from build123d import *

# Parameters (mm, degrees)
SM_BASE_FLANGE_1_DEPTH = 307.5
SKETCH_6_R             = 5.25
SKETCH_6_R_2           = 2.5
CUT_EXTRUDE_1_DEPTH    = 10
CUT_EXTRUDE_2_DEPTH    = 10
SKETCH_9_R             = 5.5
CUT_EXTRUDE_4_DEPTH    = 334.850640257
CHAMFER_1_SIZE         = 5


# Sheet-metal steps are written as plain solids
with BuildPart() as part:
    # Sketch 1 → Базовая кромка1 (new, symmetric)
    with BuildSketch(Plane.XY):
        with BuildLine():
            Line((-78, 64), (-78, 42))
            ThreePointArc((-78, 42), (-76.828427125, 39.171572875), (-74, 38))
            Line((-74, 38), (-2, 38))
            ThreePointArc((-2, 38), (-0.585786438, 37.414213562), (0, 36))
            Line((0, 36), (0, -36))
            ThreePointArc((0, -36), (-0.585786438, -37.414213562), (-2, -38))
            Line((-2, -38), (-74, -38))
            ThreePointArc((-74, -38), (-76.828427125, -39.171572875), (-78, -42))
            Line((-78, -42), (-78, -64))
            Line((-78, -64), (-76, -64))
            Line((-76, -64), (-76, -42))
            ThreePointArc((-76, -42), (-75.414213562, -40.585786438), (-74, -40))
            Line((-74, -40), (-2, -40))
            ThreePointArc((-2, -40), (0.828427125, -38.828427125), (2, -36))
            Line((2, -36), (2, 36))
            ThreePointArc((2, 36), (0.828427125, 38.828427125), (-2, 40))
            Line((-2, 40), (-74, 40))
            ThreePointArc((-74, 40), (-75.414213562, 40.585786438), (-76, 42))
            Line((-76, 42), (-76, 64))
            Line((-76, 64), (-78, 64))
        make_face()
    extrude(amount=SM_BASE_FLANGE_1_DEPTH, both=True)

    # Эскиз6 → Вырез-Вытянуть1 (cut)
    with BuildSketch(Plane(origin=(-76, 0, 0), x_dir=(0, 0, -1), z_dir=(1, 0, 0))):
        with Locations(Location((280, 55, 0), (0, 0, 90))):
            Circle(SKETCH_6_R)
        with Locations(Location((255, 55, 0), (0, 0, 90))):
            Circle(SKETCH_6_R)
        with Locations(Location((180, 57.5, 0), (0, 0, 90))):
            Circle(SKETCH_6_R_2)
        with Locations(Location((90, 57.5, 0), (0, 0, 90))):
            Circle(SKETCH_6_R_2)
        with Locations(Location((0, 57.5, 0), (0, 0, 90))):
            Circle(SKETCH_6_R_2)
        with Locations(Location((-90, 57.5, 0), (0, 0, 270))):
            Circle(SKETCH_6_R_2)
        with Locations(Location((-180, 57.5, 0), (0, 0, 270))):
            Circle(SKETCH_6_R_2)
        with Locations(Location((-255, 55, 0), (0, 0, 270))):
            Circle(SKETCH_6_R)
        with Locations(Location((-280, 55, 0), (0, 0, 270))):
            Circle(SKETCH_6_R)
    cut_extrude_1 = extrude(amount=-CUT_EXTRUDE_1_DEPTH, mode=Mode.SUBTRACT)

    # Зеркальное отражение1: Вырез-Вытянуть1 across plane
    add(cut_extrude_1.mirror(Plane.ZX), mode=Mode.SUBTRACT)

    # Эскиз7 → Вырез-Вытянуть2 (cut)
    with BuildSketch(Plane(origin=(2, 0, 0), x_dir=(0, 0, -1), z_dir=(1, 0, 0))):
        with BuildLine():
            Line((-288.5, 6.5), (-261.5, 6.5))
            ThreePointArc((-261.5, 6.5), (-255, 0), (-261.5, -6.5))
            Line((-261.5, -6.5), (-288.5, -6.5))
            ThreePointArc((-288.5, -6.5), (-295, 0), (-288.5, 6.5))
        make_face()
        with BuildLine():
            Line((-233.5, 6.5), (-206.5, 6.5))
            ThreePointArc((-206.5, 6.5), (-200, 0), (-206.5, -6.5))
            Line((-206.5, -6.5), (-233.5, -6.5))
            ThreePointArc((-233.5, -6.5), (-240, 0), (-233.5, 6.5))
        make_face()
        with BuildLine():
            Line((288.5, 6.5), (261.5, 6.5))
            ThreePointArc((261.5, 6.5), (255, 0), (261.5, -6.5))
            Line((261.5, -6.5), (288.5, -6.5))
            ThreePointArc((288.5, -6.5), (295, 0), (288.5, 6.5))
        make_face()
        with BuildLine():
            Line((233.5, 6.5), (206.5, 6.5))
            ThreePointArc((206.5, 6.5), (200, 0), (206.5, -6.5))
            Line((206.5, -6.5), (233.5, -6.5))
            ThreePointArc((233.5, -6.5), (240, 0), (233.5, 6.5))
        make_face()
    extrude(amount=-CUT_EXTRUDE_2_DEPTH, mode=Mode.SUBTRACT)

    # Эскиз9 → Вырез-Вытянуть4 (cut, through all)
    with BuildSketch(Plane(origin=(0, 40, 0), x_dir=(1, 0, 0), z_dir=(0, 1, 0))):
        with Locations(Location((-38, 0, 0), (0, 0, 270))):
            Circle(SKETCH_9_R)
    extrude(amount=-CUT_EXTRUDE_4_DEPTH, mode=Mode.SUBTRACT)

    # Фаска1
    chamfer_1_edges = [part.edges().sort_by_distance(p)[0] for p in [
        (-77, -64, -307.5),
        (-77, 64, -307.5),
        (-77, -64, 307.5),
        (-77, 64, 307.5),
    ]]
    chamfer(chamfer_1_edges, length=CHAMFER_1_SIZE)


solid = part.part
For this review, take the finished solid that the model builds, in its own axes (mm). A direction names the side the tool comes from. Coordinates: 2 decimals unless noted, no trailing zeros. Order: outer loops, then holes, each group sorted by start corner. A loop starts at its lowest first (then second) coordinate and runs counter-clockwise, first axis right, second up. Notation, with made-up numbers: (7, 0.25) - (32, 0.25) arc R18 cw to (32, 20.25) - close; hole circle Ø7 at (42, 44.25). An arc over 180 degrees is marked (long way). Answer as CSV lines item,"result". Start each with the question number.
1) Add section D-D (y = 1). State the section outline as (x, z) points.
2) Add section C-C (z = -155.5). State the section outline as (x, y) points, then the cut area to 3 significant figures.
3) Draft analysis for pull direction X (two halves, no side actions). For faces 1 (the cylindrical face through (-32.547, 39.014, -0.716)), 2 (the flat face through (0, 1, 4)), 3 (the flat face through (-31, -40, 4)), state which applies: +X half, -X half, draft (parallel to the pull), parting line (faces both ways), or undercut.
4) Add section B-B (x = -9.5). State the section outline as (y, z) points, then the cut area to 3 significant figures.
5) Machinability: for faces 4 (the cylindrical face through (-76.986, 55.683, 274.795)), 5 (the flat face through (-45, 40, 4)), 6 (the flat face through (-76, -53, 4)), which of the approach directions +Z, -Z, +X, -X, +Y, -Y give a long, thin tool a straight path to every point of the face, cutting with its end or side? Answer none if there is none.
6) Add section A-A (z = -227.5). State the section outline as (x, y) points, then the cut area to 3 significant figures.
7) Insertion check: P1, Ø8, axis at x = -31.5, z = 125, coming from the -Y side; P2, Ø4, axis at y = -40.5, z = -127.5, coming from the -X side; P3, Ø4, axis at x = -37.5, z = -104, coming from the +Y side; P4, Ø0.6, axis at x = 1, z = 279.5, coming from the -Y side. Each pin has a flat end and moves straight along its axis. Give the tip position at first contact, or say it passes through.
8) To check wall thickness, follow line 1 along Y through (x, z) = (-76.8, 90); line 2 along Y through (x, z) = (-62.5, 5); line 3 along X through (y, z) = (-14, 67.5). State the ranges of each line that lie inside material, in increasing order. Write a range as [from, to].
Result:
1,outline,"(0, -307.5) - (2, -307.5) - (2, -294.92) - (0, -294.92) - close; (0, -255.08) - (2, -255.08) - (2, -239.92) - (0, -239.92) - close; (0, -200.08) - (2, -200.08) - (2, 200.08) - (0, 200.08) - close; (0, 239.92) - (2, 239.92) - (2, 255.08) - (0, 255.08) - close; (0, 294.92) - (2, 294.92) - (2, 307.5) - (0, 307.5) - close"
2,outline,"(-78, -64) - (-76, -64) - (-76, -42) arc R2 cw to (-74, -40) - (-2, -40) arc R4 ccw to (2, -36) - (2, 36) arc R4 ccw to (-2, 40) - (-74, 40) arc R2 cw to (-76, 42) - (-76, 64) - (-78, 64) - (-78, 42) arc R4 ccw to (-74, 38) - (-2, 38) arc R2 cw to (0, 36) - (0, -36) arc R2 cw to (-2, -38) - (-74, -38) arc R4 ccw to (-78, -42) - close"
2,area,"558 mm^2"
3,face 1,"undercut"
3,face 2,"-X half"
3,face 3,"draft"
4,outline,"(-40, -307.5) - (-38, -307.5) - (-38, 307.5) - (-40, 307.5) - close; (38, -307.5) - (40, -307.5) - (40, 307.5) - (38, 307.5) - close"
4,area,"2,460 mm^2"
5,face 4,"+X, -X"
5,face 5,"+Z, -Z, +X, +Y"
5,face 6,"+Z, -Z, +X, -Y"
6,outline,"(-78, -64) - (-76, -64) - (-76, -42) arc R2 cw to (-74, -40) - (-2, -40) arc R4 ccw to (2, -36) - (2, -6.5) - (0, -6.5) - (0, -36) arc R2 cw to (-2, -38) - (-74, -38) arc R4 ccw to (-78, -42) - close; (-78, 42) arc R4 ccw to (-74, 38) - (-2, 38) arc R2 cw to (0, 36) - (0, 6.5) - (2, 6.5) - (2, 36) arc R4 ccw to (-2, 40) - (-74, 40) arc R2 cw to (-76, 42) - (-76, 64) - (-78, 64) - close"
6,area,"532 mm^2"
7,P1,"y = -40"
7,P2,"x = -78"
7,P3,"y = 40"
7,P4,"y = -38.95"
8,line 1,"[-64, -60], [-55, -39.14], [39.14, 55], [60, 64]"
8,line 2,"[-40, -38], [38, 40]"
8,line 3,"[0, 2]"
